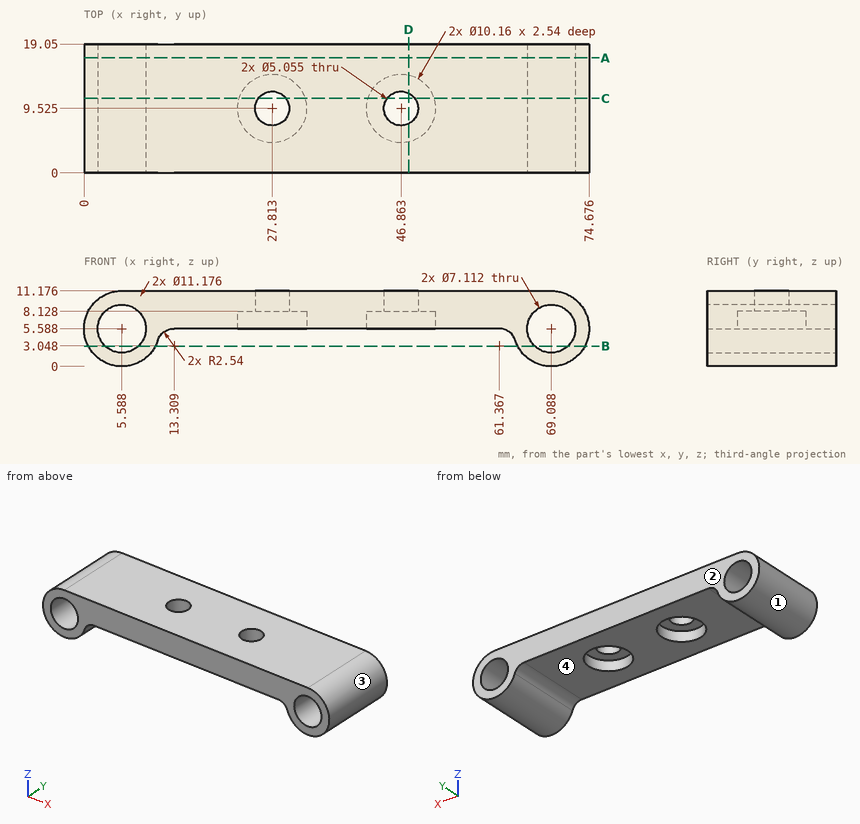
Geometry: see drawing. Coordinates: mm, zero at the bounding-box minimum. A direction names the side the tool comes from. Give positions to 0.01 mm unless a question says otherwise; leave off trailing zeros. Loops run counter-clockwise (first coordinate to the right, second up) from the corner with the lowest first, then second, coordinate; pieces in that order, holes last. Notation, with made-up numbers: (51, 32) -> (61, 32) arc R21 cw to (61, 69) -> close; hole circle Ø7 at (28.5, -17.75). An arc over 180 degrees is marked (long way). Answer as a JSON object with one key per item and string values. Group by question number.
Item 1: Cut plane A-A, the plane y = 17. Return the cut outline in (x, z), and give its area (3 significant figures).
Item 2: Cut plane C-C, the plane y = 11. Return the cut outline in (x, z) (1 decimal).
Item 3: Reachability of the marked faces 3 and 4 from +Z, -Z, +X, -X, +Y, -Y: full face, straight path, thin tool, end or side. Return the list, or none.
Item 4: Pin query (flat end, axial travel): P1, Ø5, axis at y = 11, z = 10, coming from the -X side; P2, Ø3, axis at y = 15, z = 8, coming from the +X side; P3, Ø6, axis at x = 46.863, y = 9.525, coming from the -Z side. Return the tip coordinate at first contact, or that it passes through.
Item 5: Cut plane B-B, the plane z = 3. State how many separate pieces and enclosed holes the cut face has.
Item 6: Line query: probe 1 along X at (y, z) = (13, 4) (1 decimal); probe 2 along X at (y, z) = (7.75, 6.25) (1 decimal); probe 3 along X at (y, z) = (15.5, 6) (1 decimal). Output: solid intervals per line, ascending.
Item 7: Pull-direction query (X, two-part tool) for the marked faces 1 and 2; classes: released by +X, released by -X, zero draft, split by the parting line, or undercut.
Item 8: Cut plane D-D, the plane x = 48. Return the cut outline in (y, z).
Checks:
{
 "1": {"outline": "(5.59, 11.18) arc R5.59 ccw (long way) to (10.9, 3.84) arc R2.54 cw to (13.31, 5.59) -> (61.37, 5.59) arc R2.54 cw to (63.78, 3.84) arc R5.59 ccw (long way) to (69.09, 11.18) -> close; hole circle Ø7.11 at (5.59, 5.59); hole circle Ø7.11 at (69.09, 5.59)", "area": "424 mm²"},
 "2": {"outline": "(5.6, 11.2) arc R5.6 ccw (long way) to (10.9, 3.8) arc R2.5 cw to (13.3, 5.6) -> (23, 5.6) -> (23, 8.1) -> (25.8, 8.1) -> (25.8, 11.2) -> close; (29.9, 8.1) -> (32.7, 8.1) -> (32.7, 5.6) -> (42, 5.6) -> (42, 8.1) -> (44.8, 8.1) -> (44.8, 11.2) -> (29.9, 11.2) -> close; (48.9, 8.1) -> (51.7, 8.1) -> (51.7, 5.6) -> (61.4, 5.6) arc R2.5 cw to (63.8, 3.8) arc R5.6 ccw (long way) to (69.1, 11.2) -> (48.9, 11.2) -> close; hole circle Ø7.1 at (5.6, 5.6); hole circle Ø7.1 at (69.1, 5.6)"},
 "3": {"face 3": "+Y, -Y", "face 4": "-Z, +Y, -Y"},
 "4": {"P1": "stops at x = 0.34", "P2": "stops at x = 74.6", "P3": "stops at z = 8.13"},
 "5": {"separate pieces": "4", "enclosed holes": "0"},
 "6": {"probe 1": "x = 0.2 to 2.4, 8.8 to 11, 63.7 to 65.9, 72.3 to 74.4", "probe 2": "x = 0 to 2.1, 9.1 to 23.1, 32.6 to 42.1, 51.6 to 65.6, 72.6 to 74.6", "probe 3": "x = 0 to 2.1, 9.1 to 65.6, 72.6 to 74.7"},
 "7": {"face 1": "undercut", "face 2": "zero draft"},
 "8": {"outline": "(0, 5.59) -> (4.57, 5.59) -> (4.57, 8.13) -> (7.27, 8.13) -> (7.27, 11.18) -> (0, 11.18) -> close; (11.78, 8.13) -> (14.48, 8.13) -> (14.48, 5.59) -> (19.05, 5.59) -> (19.05, 11.18) -> (11.78, 11.18) -> close"}
}
